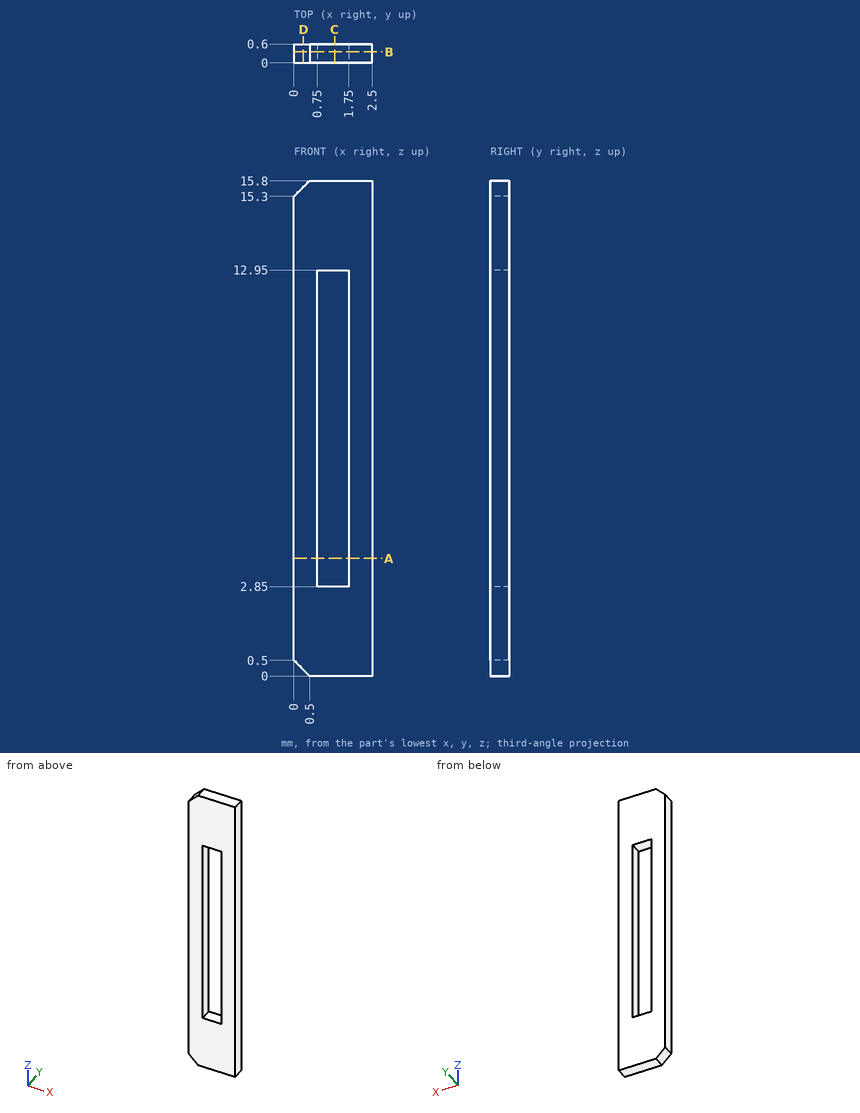
Source: three-view drawing plus pictorial views. Frame: mm from the lowest corner of the part. Round coordinates to 2 decimals unless told otherwise and drop trailing zeros. Loops run counter-clockwise (first coordinate to the right, second up) from the corner with the lowest first, then second, coordinate; pieces in that order, holes last.
Q1. Section A-A on z = 3.75. Return loops of the section in (x, y), plus the area to 3 significant figures.
Q2. Material intervals for L1, parallel to X at y = 0.35, z = 4.5; L2, parallel to Z at x = 1.3, y = 0.1; L3, parallel to Z at x = 0.35, y = 0.15, sorted ascending.
Q3. Section B-B on y = 0.35. Return loops of the section in (x, z).
Q4. Section C-C on x = 1.3. Return loops of the section in (y, z).
Q5. Section D-D on x = 0.3. Return loops of the section in (y, z).
Q6. Pin query (flat end, axial travel): P1, Ø1.5, axis at x = 1.5, z = 8, coming from the +Y side. Return the tip coordinate at first contact, or that it passes through.
Evaluation:
1. outline: (0, 0) - (0.75, 0) - (0.75, 0.6) - (0, 0.6) - close; (1.75, 0) - (2.5, 0) - (2.5, 0.6) - (1.75, 0.6) - close
1. area: 0.900 mm2
2. L1: x = 0 to 0.75, 1.75 to 2.5
2. L2: z = 0 to 2.85, 12.95 to 15.8
2. L3: z = 0.15 to 15.65
3. outline: (0, 0.5) - (0.5, 0) - (2.5, 0) - (2.5, 15.8) - (0.5, 15.8) - (0, 15.3) - close; hole (0.75, 2.85) - (1.75, 2.85) - (1.75, 12.95) - (0.75, 12.95) - close
4. outline: (0, 0) - (0.6, 0) - (0.6, 2.85) - (0, 2.85) - close; (0, 12.95) - (0.6, 12.95) - (0.6, 15.8) - (0, 15.8) - close
5. outline: (0, 0.2) - (0.6, 0.2) - (0.6, 15.6) - (0, 15.6) - close
6. P1: stops at y = 0.6
